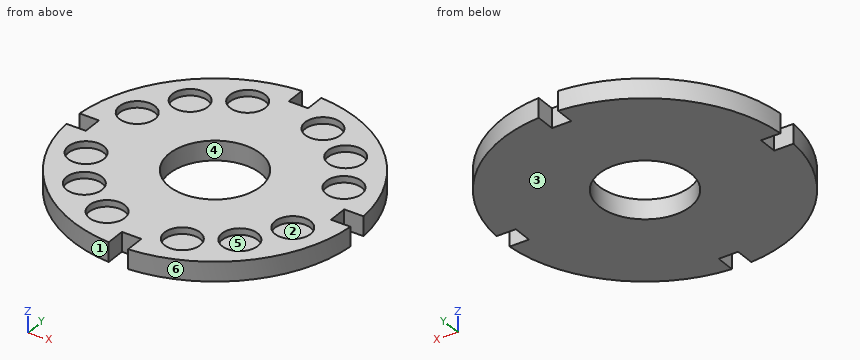
from build123d import *

# Parameters (mm, degrees)
F0_R            = 44.8437
F0_R_2          = 17.4625
F0_W            = 19.05
F0_H            = 6.35
F1_DEPTH        = 19.05
F2_DEPTH        = 6.35
F2_COPIES_COUNT = 4
F3_DEPTH        = 19.051
F3_COPIES_COUNT = 4
F5_DEPTH        = 25.4


# Not quite as in the source:
# - a pattern or mirror of a feature is missing from the dataset's text; its kind, count and spacing are read off the source's solid


with BuildPart() as f1:
    # F0 (on Top) → F1 (new body)
    with BuildSketch(Plane.XY):
        with BuildLine():
            ThreePointArc((-9.525, 139.3749058296), (-95.3557746023, -102.0948884617), (139.7, 0))
            ThreePointArc((139.7, 0), (102.0948884617, 95.3557746023), (9.525, 139.3749058296))
            Line((9.525, 139.3749058296), (9.525, 120.3249058296))
            Line((9.525, 120.3249058296), (9.525, 113.9749058296))
            Line((9.525, 113.9749058296), (-9.525, 113.9749058296))
            Line((-9.525, 113.9749058296), (-9.525, 120.3249058296))
            Line((-9.525, 120.3249058296), (-9.525, 139.3749058296))
        make_face()
        Circle(F0_R, mode=Mode.SUBTRACT)
        with Locations((101.4398184138, 36.921074472)):
            Circle(F0_R_2, mode=Mode.SUBTRACT)
        with Locations((36.921074472, 101.4398184138)):
            Circle(F0_R_2, mode=Mode.SUBTRACT)
        with Locations((76.3321770291, 76.3321770291)):
            Circle(F0_R_2, mode=Mode.SUBTRACT)
        with BuildLine():
            Line((9.525, 120.3249058296), (9.525, 139.3749058296))
            ThreePointArc((9.525, 139.3749058296), (0, 139.7), (-9.525, 139.3749058296))
            Line((-9.525, 139.3749058296), (-9.525, 120.3249058296))
            Line((-9.525, 120.3249058296), (9.525, 120.3249058296))
        make_face()
        with Locations((36.921074472, 101.4398184138)):
            Circle(F0_R_2)
        with Locations((76.3321770291, 76.3321770291)):
            Circle(F0_R_2)
        with Locations((101.4398184138, 36.921074472)):
            Circle(F0_R_2)
        with Locations((0, 117.1499058296)):
            Rectangle(F0_W, F0_H)
        Circle(F0_R)
    extrude(amount=-F1_DEPTH)

    # F0 (on Top) → F2 (cut)
    with BuildSketch(Plane.XY):
        with Locations((36.921074472, 101.4398184138)):
            Circle(F0_R_2)
        with Locations((76.3321770291, 76.3321770291)):
            Circle(F0_R_2)
        with Locations((101.4398184138, 36.921074472)):
            Circle(F0_R_2)
    f2 = extrude(amount=-F2_DEPTH, mode=Mode.SUBTRACT)

    # F2_copies: F2 ×4 about axis
    f2_copies_axis = Axis((0, 0, 0), (0, 0, 1))
    for i in range(1, F2_COPIES_COUNT):
        add(f2.rotate(f2_copies_axis, i * 360 / F2_COPIES_COUNT), mode=Mode.SUBTRACT)

    # F0 (on Top) → F3 (cut, through all)
    with BuildSketch(Plane.XY):
        with BuildLine():
            Line((9.525, 120.3249058296), (9.525, 139.3749058296))
            ThreePointArc((9.525, 139.3749058296), (0, 139.7), (-9.525, 139.3749058296))
            Line((-9.525, 139.3749058296), (-9.525, 120.3249058296))
            Line((-9.525, 120.3249058296), (9.525, 120.3249058296))
        make_face()
    f3 = extrude(amount=-F3_DEPTH, mode=Mode.SUBTRACT)

    # F3_copies: F3 ×4 about axis
    f3_copies_axis = Axis((0, 0, 0), (0, 0, 1))
    for i in range(1, F3_COPIES_COUNT):
        add(f3.rotate(f3_copies_axis, i * 360 / F3_COPIES_COUNT), mode=Mode.SUBTRACT)

    # F0 (on Top) → F5 (cut)
    with BuildSketch(Plane.XY):
        Circle(F0_R)
    extrude(amount=-F5_DEPTH, mode=Mode.SUBTRACT)


solid = f1.part
Can you work these out from the model? Positions are in its coordinate system, mm. Face numbers are marked on the shaded views. A direction names the side the tool comes from. Give positions to 0.01 mm unless a question says otherwise; leave off trailing zeros. Order: outer loops, then holes, each group sorted by start corner. A loop starts at its lowest first (then second) coordinate and runs counter-clockwise, first axis right, second up. Notation, with made-up numbers: (78, 34.25) - (136, 34.25) arc R18 ccw to (136, 51.25) - close; hole circle Ø9 at (9, 29). An arc over 180 degrees is marked (long way). Write each question's results on one line, items separated by ' | '.
1) Suppose I cut it at B-B, the plane z = -11.25. Write out the boundary of the cut face in (x, y) (3 decimals), then the cut area to 3 significant figures.
Final values:
outline: (-139.375, -9.525) arc R139.7 ccw to (-9.525, -139.375) - (-9.525, -120.325) - (9.525, -120.325) - (9.525, -139.375) arc R139.7 ccw to (139.375, -9.525) - (120.325, -9.525) - (120.325, 9.525) - (139.375, 9.525) arc R139.7 ccw to (9.525, 139.375) - (9.525, 120.325) - (-9.525, 120.325) - (-9.525, 139.375) arc R139.7 ccw to (-139.375, 9.525) - (-120.325, 9.525) - (-120.325, -9.525) - close; hole circle Ø89.687 at (0, 0) | area: 53,500 mm^2
2) Please list where these lines run through material, in increasing order: line 1 along X through (y, z) = (-77.5, -2); line 2 along X through (y, z) = (114, -4); line 3 along Y through (x, z) = (-40.5, -1). Write a range as [from, to].
Final values:
line 1: x = [-116.23, -93.76], [-58.91, 58.91], [93.76, 116.23] | line 2: x = [-80.75, -49.05], [-24.79, 24.79], [49.05, 80.75] | line 3: y = [-133.7, -118.53], [-84.35, -19.25], [19.25, 84.35], [118.53, 133.7]
3) If we mould it in two halves opening along X, with no side actions, what happens to the marked faces 1, 2, 3 and 4? For each: pulls with the +X half, pulls with the -X half, needs draft (parallel to the pull), parting line crosses it, or undercut.
Final values:
face 1: pulls with the -X half | face 2: undercut | face 3: needs draft | face 4: undercut
4) I'm going to push flat-ended pins straight in: pin 1 Ø5.5 at (y, z) = (-1.5, -10) entering from +X; pin 2 Ø10.5 at (x, y) = (74.5, -75.5) entering from +Z; pin 3 Ø3 at (y, z) = (-81, -2) entering from +X. Where does each tip first touch, or does it pass through?
Final values:
pin 1: stops at x = 120.32 | pin 2: stops at z = -6.35 | pin 3: stops at x = 114.87
5) Suppose I cut it at A-A, the plane y = 0. Write out the boundary of the cut face in (x, z).
Final values:
outline: (-120.32, -19.05) - (-44.84, -19.05) - (-44.84, 0) - (-120.32, 0) - close; (44.84, -19.05) - (120.32, -19.05) - (120.32, 0) - (44.84, 0) - close
6) On a 3-axis mill with a long thin cutter (end or side, diameter ignored), from which of +Z, -Z, +X, -X, +Y, -Y can I reach the whole of each face in a straight line? I mean the marked faces 5 and 6. Say none if no direction works.
Final values:
face 5: +Z | face 6: +Z, -Z, +X, -Y
7) Suppose I cut it at D-D, the plane x = 107. Write out the boundary of the cut face in (y, z).
Final values:
outline: (-89.82, -19.05) - (89.82, -19.05) - (89.82, 0) - (53.47, 0) - (53.47, -6.35) - (20.37, -6.35) - (20.37, 0) - (-20.37, 0) - (-20.37, -6.35) - (-53.47, -6.35) - (-53.47, 0) - (-89.82, 0) - close
